Verification items for the finished model (mm, model axes). A direction names the side the tool comes from. Coordinates: 2 decimals unless noted, no trailing zeros. Order: outer loops, then holes, each group sorted by start corner. A loop starts at its lowest first (then second) coordinate and runs counter-clockwise, first axis right, second up. Notation, with made-up numbers: M 17,58 L 46,58 A17 cw 46,79 Z; hole C 79.25,-15 d5. An arc over 180 degrees is marked long. Answer as a JSON object with one key per item and string values. Group by question number.
(1) Mould release check, pull along X, two halves, no side actions. Record for faces 1 (the face through (111.37, 55.61, -6.2)), 2 (the face through (88, 106.103, 14)), 3 (the face through (115.43, 80.75, 12.81)), 4 (the face through (95.96, 55.61, 9.21)): released by +X, released by -X, zero draft, split by the parting line, or undercut.
(2) Cross-section at B-B (y = 48.5). Enter the section's corners in (x, z).
(3) Cross-section at C-C (y = 71). Enter the section's corners in (x, z), plus the area to 3 significant figures.
(4) Gauge pin test, flat ends, axial feed: pin 1 Ø2 at (x, z) = (113.5, -9.5) entering from -Y; pin 2 Ø9 at (x, y) = (102.5, 38.5) entering from +Z; pin 3 Ø4 at (x, y) = (101.5, 35.5) entering from -Z. Record the tip position at first contact, or that the pin passes through.
(5) Material ranges on line 1 (Y direction, x = 102.5, z = -6); line 2 (Y direction, x = 106.5, z = 5.5); line 3 (Z direction, x = 101.5, y = 56), recorded low to high.
(6) Access from +Z, -Z, +X, -X, +Y, -Y to the whole of each face (thin tool, end or side, straight path). Record for faces 5 (the face through (106, 33, -2.5)), 6 (the face through (106, 33, 2.5)), 7 (the face through (104.1, 34.7, 8.5)), 8 (the face through (89.828, 80.753, 13.805)).
(7) Cross-section at A-A (z = 14). Enter the section's corners in (x, y).
from build123d import *
from build123d.topology import SkipClean

# Parameters (mm, degrees)
SKETCH1_R                           = 7.5
SKETCH1_R_2                         = 2.05
BOSS_EXTRUDE1_DEPTH                 = 2.5
SKETCH2_R                           = 4
SKETCH2_R_2                         = 2.05
BOSS_EXTRUDE2_DEPTH                 = 6
SKETCH7_W                           = 4
SKETCH7_H                           = 18.687164731
REVOLVE7_ANGLE                      = 180
SKETCH8_W                           = 2.05
SKETCH8_H                           = 18.687164731
SKETCH9_R                           = 2.05
CUT_EXTRUDE1_DEPTH                  = 5
BOSS_EXTRUDE3_START                 = 1
SKETCH10_R                          = 2.05
BOSS_EXTRUDE3_DEPTH                 = 1
SKETCH11_R                          = 1.5
BOSS_EXTRUDE4_DEPTH                 = 50
M3X0_5_TAPPED_HOLE1_REACH           = 76.406
M3X0_5_TAPPED_HOLE1_BORE_R          = 1.25
M3X0_5_TAPPED_HOLE1_ON_FACE_2_REACH = 76.436
M3X0_5_TAPPED_HOLE1_BORE_2_R        = 1.25


with BuildPart() as part:
    # Sketch1 → Boss-Extrude1 (new body)
    with BuildSketch(Plane.XY):
        with Locations((102.341205301, 36.416113389)):
            Circle(SKETCH1_R)
        with Locations((102.341205301, 36.416113389)):
            Circle(SKETCH1_R_2, mode=Mode.SUBTRACT)
    boss_extrude1 = extrude(amount=BOSS_EXTRUDE1_DEPTH)

    # Sketch2 → Boss-Extrude2 (add)
    with BuildSketch(Plane.XY.offset(2.5)):
        with Locations((102.341205301, 36.416113389)):
            Circle(SKETCH2_R)
        with Locations((102.341205301, 36.416113389)):
            Circle(SKETCH2_R_2, mode=Mode.SUBTRACT)
    boss_extrude2 = extrude(amount=BOSS_EXTRUDE2_DEPTH)

    # Sketch7 → Revolve7 (revolve)
    with BuildSketch(Plane(origin=(0, 0, 0), x_dir=(-1, 0, 0), z_dir=(0, 0, -1))):
        with Locations((-104.341205301, 45.759695755)):
            Rectangle(SKETCH7_W, SKETCH7_H)
    revolve7 = revolve(axis=Axis((102.341205301, 36.416113389, 0), (0, -1, 0)), revolution_arc=REVOLVE7_ANGLE)

    # Sketch8 → Cut-Revolve2 (revolve, cut)
    with BuildSketch(Plane(origin=(0, 0, 0), x_dir=(-1, 0, 0), z_dir=(0, 0, -1))):
        with Locations((-103.366205301, 45.759695755)):
            Rectangle(SKETCH8_W, SKETCH8_H)
    cut_revolve2 = revolve(axis=Axis((102.341205301, 36.416113389, 0), (0, 1, 0)), mode=Mode.SUBTRACT)

    # Sketch9 → Cut-Extrude1 (cut)
    with SkipClean():  # the faces are left unmerged after this step: merging them gives an invalid solid
        with BuildSketch(Plane(origin=(0, 0, 0), x_dir=(-1, 0, 0), z_dir=(0, 0, -1))):
            with Locations(Location((-102.341205301, 36.416113389, 0), (0, 0, 180))):
                Circle(SKETCH9_R)
        cut_extrude1 = extrude(amount=-CUT_EXTRUDE1_DEPTH, mode=Mode.SUBTRACT)

    # Mirror1: Boss-Extrude1, Boss-Extrude2, Revolve7, Cut-Revolve2, Cut-Extrude1 across plane
    with SkipClean():  # the faces are left unmerged after this step: merging them gives an invalid solid
        add(boss_extrude1.mirror(Plane(origin=(102.341205301, 36.416113389, 0), x_dir=(1, 0, 0), z_dir=(0, 0, 1))))
        add(boss_extrude2.mirror(Plane(origin=(102.341205301, 36.416113389, 0), x_dir=(1, 0, 0), z_dir=(0, 0, 1))))
        add(revolve7.mirror(Plane(origin=(102.341205301, 36.416113389, 0), x_dir=(1, 0, 0), z_dir=(0, 0, 1))))
        add(cut_revolve2.mirror(Plane(origin=(102.341205301, 36.416113389, 0), x_dir=(1, 0, 0), z_dir=(0, 0, 1))), mode=Mode.SUBTRACT)
        add(cut_extrude1.mirror(Plane(origin=(102.341205301, 36.416113389, 0), x_dir=(1, 0, 0), z_dir=(0, 0, 1))), mode=Mode.SUBTRACT)

    # Sketch10 → Boss-Extrude3 (add)
    with BuildSketch(Plane(origin=(0, 55.10327812, 0), x_dir=(1, 0, 0), z_dir=(0, 1, 0)).offset(BOSS_EXTRUDE3_START)):
        with BuildLine():
            Line((102.341205301, 2.828427125), (89.755418863, 15.414213562))
            ThreePointArc((89.755418863, 15.414213562), (86.926991738, 15.414213562), (86.926991738, 12.585786438))
            Line((86.926991738, 12.585786438), (99.512778176, 0))
            Line((99.512778176, 0), (86.926991738, -12.585786438))
            ThreePointArc((86.926991738, -12.585786438), (86.926991738, -15.414213562), (89.755418863, -15.414213562))
            Line((89.755418863, -15.414213562), (102.341205301, -2.828427125))
            Line((102.341205301, -2.828427125), (114.926991738, -15.414213562))
            ThreePointArc((114.926991738, -15.414213562), (117.755418863, -15.414213562), (117.755418863, -12.585786438))
            Line((117.755418863, -12.585786438), (105.169632425, 0))
            Line((105.169632425, 0), (117.755418863, 12.585786438))
            ThreePointArc((117.755418863, 12.585786438), (117.755418863, 15.414213562), (114.926991738, 15.414213562))
            Line((114.926991738, 15.414213562), (102.341205301, 2.828427125))
        make_face()
        with Locations(Location((102.341205301, 0, 0), (0, 0, 180))):
            Circle(SKETCH10_R, mode=Mode.SUBTRACT)
    extrude(amount=-BOSS_EXTRUDE3_DEPTH)

    # Sketch11 → Boss-Extrude4 (add)
    with BuildSketch(Plane(origin=(0, 56.10327812, 0), x_dir=(1, 0, 0), z_dir=(0, 1, 0))):
        with Locations(Location((88.341205301, 14, 0), (0, 0, 270))):
            Circle(SKETCH11_R)
        with Locations(Location((116.341205301, 14, 0), (0, 0, 270))):
            Circle(SKETCH11_R)
        with Locations(Location((116.341205301, -14, 0), (0, 0, 270))):
            Circle(SKETCH11_R)
        with Locations(Location((88.341205301, -14, 0), (0, 0, 270))):
            Circle(SKETCH11_R)
    extrude(amount=BOSS_EXTRUDE4_DEPTH)

    # M3x0.5 Tapped Hole1 bore (on position points) → M3x0.5 Tapped Hole1 (cut, up to next)
    with BuildSketch(Plane(origin=(98.587954415, 37.799264786, 5.923678009), x_dir=(-0.345787849288, -0.938312721477, 0), z_dir=(-0.938312721477, 0.345787849288, 0)), mode=Mode.PRIVATE) as m3x0_5_tapped_hole1_sk1:
        Circle(M3X0_5_TAPPED_HOLE1_BORE_R)
    m3x0_5_tapped_hole1_tool1 = extrude(m3x0_5_tapped_hole1_sk1.sketch, amount=-M3X0_5_TAPPED_HOLE1_REACH, mode=Mode.PRIVATE) & part.part
    add(m3x0_5_tapped_hole1_tool1.solids().sort_by_distance((98.587954, 37.799265, 5.923678))[0], mode=Mode.SUBTRACT)

    # M3x0.5 Tapped Hole1 bore 2 (on position points) → M3x0.5 Tapped Hole1 on face 2 (cut, up to next)
    with BuildSketch(Plane(origin=(98.537036141, 37.652356489, -5.51866452), x_dir=(-0.309061063746, -0.95104219616, 0), z_dir=(-0.95104219616, 0.309061063746, 0)), mode=Mode.PRIVATE) as m3x0_5_tapped_hole1_on_face_2_sk1:
        Circle(M3X0_5_TAPPED_HOLE1_BORE_2_R)
    m3x0_5_tapped_hole1_on_face_2_tool1 = extrude(m3x0_5_tapped_hole1_on_face_2_sk1.sketch, amount=-M3X0_5_TAPPED_HOLE1_ON_FACE_2_REACH, mode=Mode.PRIVATE) & part.part
    add(m3x0_5_tapped_hole1_on_face_2_tool1.solids().sort_by_distance((98.537036, 37.652356, -5.518665))[0], mode=Mode.SUBTRACT)


solid = part.part
Taken from the geometry:
{
 "1": {"face 1": "released by +X", "face 2": "zero draft", "face 3": "undercut", "face 4": "undercut"},
 "2": {"outline": "C 102.34,0 d8; hole C 102.34,0 d4.1"},
 "3": {"outline": "C 88.34,-14 d3; C 88.34,14 d3; C 116.34,-14 d3; C 116.34,14 d3", "area": "28.3 mm²"},
 "4": {"pin 1": "stops at y = 55.1", "pin 2": "stops at z = 8.5", "pin 3": "stops at z = -8.5"},
 "5": {"line 1": "y = 32.42 to 34.37, 38.46 to 40.41", "line 2": "y = 55.1 to 56.1", "line 3": "z = -3.67 to -1.87, 1.87 to 3.67"},
 "6": {"face 5": "-Z", "face 6": "+Z", "face 7": "+Z, +X, -X, +Y, -Y", "face 8": "+Y"},
 "7": {"outline": "M 86.34,55.1 L 91.17,55.1 L 91.17,56.1 L 89.84,56.1 L 89.84,106.1 L 86.84,106.1 L 86.84,56.1 L 86.34,56.1 Z; M 113.51,55.1 L 118.34,55.1 L 118.34,56.1 L 117.84,56.1 L 117.84,106.1 L 114.84,106.1 L 114.84,56.1 L 113.51,56.1 Z"}
}
